Drawing for the job (mm, zero at the part's lowest x, y, z). A direction names the side the tool comes from. Coordinates: 2 decimals unless noted, no trailing zeros. Write each loop counter-clockwise with the first axis right and the second up, starting at its lowest first coordinate (ties: lowest second). Pieces come first, ordered by that corner, then holes. Notation, with made-up numbers: M 29.25,24 L 87.25,24 A13 ccw 87.25,39 Z; hole C -36.75,-25 d4. An arc over 180 degrees is marked long. Use a Markdown table: item, result. Add a question column.
Q1. Wall check: L1, parallel to Y at x = 99, z = 10; L2, parallel to X at y = 16, z = 7; L3, parallel to X at y = 13.5, z = 3.5. Give the ranges that are in metal, low to high. Write a range as from..to.
Q2. Slice it at B-B on x = 95. Write the cut outline in (y, z).
Q3. Slice it at C-C on z = 12.25. Write the cut outline in (x, y), then the cut area to 3 significant figures.
Q4. Tool access for the marked faces 1, 2 and 3: list every direction of +Z, -Z, +X, -X, +Y, -Y with a clear straight run to the whole face (end or side of a thin tool).
Q5. Mould opens along X. For the marked faces 4, 5 and 6 say: released by +X, released by -X, zero draft, split by the parting line, or undercut.
Q6. Slice it at D-D on x = 31. Write the cut outline in (y, z), then the cut area to 3 significant figures.
Q7. Slice it at A-A on y = 18. Write the cut outline in (x, z).
Q8. Pin check, flat tips, straight feed: pin 1 Ø12 at (x, z) = (49, 8) entering from -Y; pin 2 Ø4 at (y, z) = (15, 18.5) entering from +X; pin 3 Ø6 at (x, y) = (88.5, 4) entering from +Z; pin 4 Ø1 at (x, z) = (86.5, 4) entering from +Y. Stop position of each tip, or through.
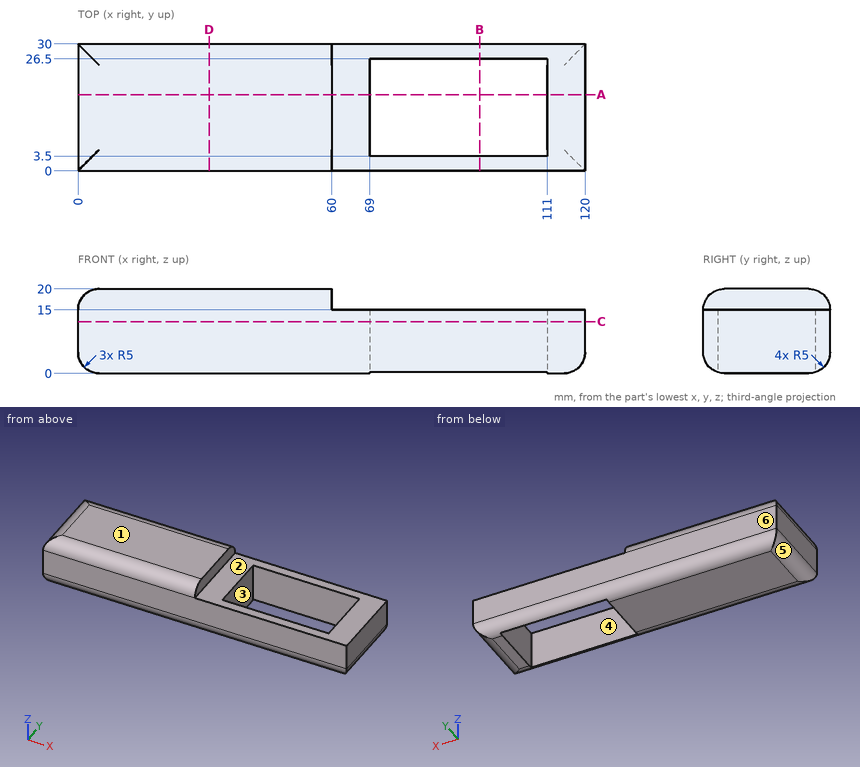
Recorded:
| question | item | result |
|---|---|---|
| 1 | L1 | 0..3.5, 26.5..30 |
| 1 | L2 | 0..69, 111..120 |
| 1 | L3 | 0.23..69, 111..119.77 |
| 2 | outline | M 0,5 A5 ccw 3.5,0.23 L 3.5,15 L 0,15 Z; M 26.5,0.23 A5 ccw 30,5 L 30,15 L 26.5,15 Z |
| 3 | outline | M 0,0 L 120,0 L 120,30 L 0,30 Z; hole M 69,3.5 L 111,3.5 L 111,26.5 L 69,26.5 Z |
| 3 | area | 2,630 mm² |
| 4 | face 1 | +Z, +X, -X, +Y, -Y |
| 4 | face 2 | +Z, +X, +Y, -Y |
| 4 | face 3 | +Z, -Z |
| 5 | face 4 | undercut |
| 5 | face 5 | released by -X |
| 5 | face 6 | zero draft |
| 6 | outline | M 0,5 A5 ccw 5,0 L 25,0 A5 ccw 30,5 L 30,15 A5 ccw 25,20 L 5,20 A5 ccw 0,15 Z |
| 6 | area | 579 mm² |
| 7 | outline | M 0,5 A5 ccw 5,0 L 69,0 L 69,15 L 60,15 L 60,20 L 5,20 A5 ccw 0,15 Z; M 111,0 L 115,0 A5 ccw 120,5 L 120,15 L 111,15 Z |
| 8 | pin 1 | y = 0 |
| 8 | pin 2 | x = 60 |
| 8 | pin 3 | z = 15 |
| 8 | pin 4 | y = 29.97 |
